Geometry check sheet. Reference: the model listing, model coordinates, mm. A direction names the side the tool comes from. Coordinates: 2 decimals unless noted, no trailing zeros. Write each loop counter-clockwise with the first axis right and the second up, starting at its lowest first coordinate (ties: lowest second). Pieces come first, ordered by that corner, then holes. Notation, with made-up numbers: (57.25, 2) -> (83.25, 2) arc R8 cw to (83.25, 9) -> close; hole circle Ø6 at (15, 81.25). An arc over 180 degrees is marked (long way). Use a Markdown table: item, result.
```python
from build123d import *

# Parameters (mm, degrees)
CHAMFER1_SIZE = 0.635


with BuildPart() as part:
    # Sketch1 → Revolve1 (revolve)
    with BuildSketch(Plane.XY):
        Polygon((-9.5631, 24.49576), (-9.5631, 45.33392), (-7.366, 45.33392), (-7.366, 47.49292), (-9.5631, 47.49292), (-9.5631, 48.76292), (-6.35, 48.76292), (-6.35, 0), (-9.5631, 0), (-9.5631, 1.27), (-8.9408, 1.27), (-8.9408, 2.4384), (-9.5631, 2.4384), (-9.5631, 23.07336), (-8.8011, 23.07336), (-8.8011, 24.49576), align=None)
    revolve(axis=Axis((0, 55, 0), (0, -1, 0)))

    # Chamfer1
    chamfer1_edges = [part.edges().sort_by_distance(p)[0] for p in [
        (9.5631, 0, 0),
        (9.5631, 48.76292, 0),
    ]]
    chamfer(chamfer1_edges, length=CHAMFER1_SIZE)


solid = part.part
```
Item 1: Tool access check on faces 1 (the cylindrical face through (-9.121, 0.957, -2.872)), 2 (the cylindrical face through (-3.399, 46.429, 6.535)). Record the directions out of +Z, -Z, +X, -X, +Y, -Y that give a thin tool (end or side, any length) a straight path to the whole face; none if there is none.
Answer block:
| item | result |
|---|---|
| face 1 | +Y, -Y |
| face 2 | none |
Item 2: Depth check by flat-ended pin: P1, Ø6, axis at y = 34, z = 5, coming from the -X side; P2, Ø5.5, axis at x = -4.5, z = 1.5, coming from the -Y side; P3, Ø4, axis at y = 9.5, z = 5.5, coming from the -X side; P4, Ø5, axis at x = 5.5, y = 18, coming from the -Z side. Enter the tip coordinate at first touch or a pass-through.
Answer block:
| item | result |
|---|---|
| P1 | stops at x = -9.35 |
| P2 | stops at y = 0 |
| P3 | stops at x = -8.9 |
| P4 | stops at z = -9.08 |
Item 3: Thickness scan on L1, parallel to X at y = 26.5, z = 0; L2, parallel to Y at x = 3.75, z = -6.75. Record the ranges inside material, lowest first. Write a range as [from, to].
Answer block:
| item | result |
|---|---|
| L1 | x = [-9.56, -6.35], [6.35, 9.56] |
| L2 | y = [0, 45.33], [47.49, 48.76] |
Item 4: Mould release check, pull along Y, two halves, no side actions. Record for faces 3 (the cylindrical face through (-9.121, 35.061, -2.872)), 4 (the flat face through (6.33, 24.496, 6.33)), 5 (the flat face through (4, 0, 6)): +Y half, -Y half, draft (parallel to the pull), parting line (faces both ways), or undercut.
Answer block:
| item | result |
|---|---|
| face 3 | draft |
| face 4 | undercut |
| face 5 | -Y half |
Item 5: Section check A-A on y = 3. Record the boundary of the cut face in (x, z), then the cut area to 3 significant figures.
Answer block:
| item | result |
|---|---|
| outline | circle Ø19.13 at (0, 0); hole circle Ø12.7 at (0, 0) |
| area | 161 mm^2 |
